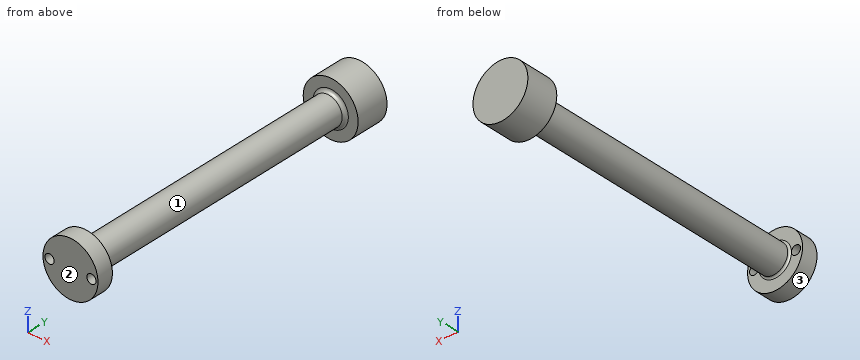
from build123d import *

# Parameters (mm, degrees)
SKETCH2_R          = 1.7779999999999996
CUT_EXTRUDE1_DEPTH = 6.35
FILLET1_R          = 1.27
FILLET2_R          = 0.762


with BuildPart() as part:
    # Sketch1 → Revolve1 (revolve)
    with BuildSketch(Plane.XY, mode=Mode.PRIVATE) as revolve1_sk:
        Polygon((0, 0), (10.668, 0), (10.668000000000001, 6.35), (5.588, 6.349999999999999), (5.588, 114.30000000000001), (10.668000000000001, 114.3), (10.668, 127), (-1.12e-14, 127), align=None)
    revolve(revolve1_sk.sketch.rotate(Axis((-1.12e-14, 127, 0), (9e-17, -1, 0)), 180), axis=Axis((-1.12e-14, 127, 0), (9e-17, -1, 0)))

    # Sketch2 → Cut-Extrude1 (cut)
    with BuildSketch(Plane(origin=(-5.6e-16, 6.349999999999999, 0), x_dir=(1, -1.7e-16, 0), z_dir=(1.7e-16, 1, 0))):
        with Locations(Location((-8.128000000000021, -4.5e-16, 0), (0, 0, 180))):
            Circle(SKETCH2_R)
        with Locations(Location((8.128000000000021, -4.5e-16, 0), (0, 0, 180))):
            Circle(SKETCH2_R)
    extrude(amount=-CUT_EXTRUDE1_DEPTH, mode=Mode.SUBTRACT)

    # Fillet1
    fillet1_edges = [part.edges().sort_by_distance(p)[0] for p in [
        (5.588000000000001, 114.30000000000001, -1.37e-15),
    ]]
    fillet(fillet1_edges, radius=FILLET1_R)

    # Fillet2
    fillet2_edges = [part.edges().sort_by_distance(p)[0] for p in [
        (5.587999999999999, 6.349999999999995, -3.85e-15),
    ]]
    fillet(fillet2_edges, radius=FILLET2_R)


solid = part.part
Could you check a few things on this model? Use its own coordinates, in mm. Face numbers are marked on the shaded views. Coordinates: 2 decimals unless noted, no trailing zeros. Order: outer loops, then holes, each group sorted by start corner. A loop starts at its lowest first (then second) coordinate and runs counter-clockwise, first axis right, second up. Notation, with made-up numbers: (10.25, 69) - (25.25, 69) arc R20 ccw to (25.25, 75) - close; hole circle Ø10 at (8.5, 48). An arc over 180 degrees is marked (long way). Answer in a Markdown table with one row per item. Add a question column.
(1) Will these pins go through, and if not, where does the flat tip stop? pin 1 (10 mm diameter, centred on x = 8.5, z = 0.5, fed in from -Y); pin 2 (10 mm diameter, centred on x = -2, y = 51, fed in from +Z); pin 3 (3 mm diameter, centred on x = -8.128, z = 0, fed in from -Y); pin 4 (10 mm diameter, centred on x = 6, y = 106, fed in from +Z).
(2) I need wall thicknesses on L1, parallel to Y at x = -0.5, z = -9; L2, parallel to Z at x = 1.5, y = 87; L3, parallel to Y at x = -6, z = 0.5. Which ranges of each line are inside material? Lowest first, please.
(3) If we section it at A-A, the plane x = 0: Please give me the cut outline in (y, z), then the cut area to 3 significant figures.
(4) If we section it at B-B, the plane z = -8.25: Please give me the cut outline in (x, y).
(5) If we mould it in two halves opening along Y, with no side actions, what happens to the marked faces 1, 2 and 3? For each: released by +Y, released by -Y, zero draft, split by the parting line, or undercut.
(6) If we section it at D-D, the plane z = 9: Please give me the cut outline in (x, y), then the cut area to 3 significant figures.
(7) If we section it at C-C, the plane y = 99: Please give me the cut outline in (x, z).
Results are:
| question | item | result |
|---|---|---|
| 1 | pin 1 | stops at y = 0 |
| 1 | pin 2 | stops at z = 5.59 |
| 1 | pin 3 | stops at y = 114.28 |
| 1 | pin 4 | stops at z = 5.5 |
| 2 | L1 | y = 0 to 6.35, 114.3 to 127 |
| 2 | L2 | z = -5.38 to 5.38 |
| 2 | L3 | y = 0 to 6.42, 113.98 to 127 |
| 3 | outline | (0, -10.67) - (6.35, -10.67) - (6.35, -6.35) arc R0.76 cw to (7.11, -5.59) - (113.03, -5.59) arc R1.27 cw to (114.3, -6.86) - (114.3, -10.67) - (127, -10.67) - (127, 10.67) - (114.3, 10.67) - (114.3, 6.86) arc R1.27 cw to (113.03, 5.59) - (7.11, 5.59) arc R0.76 cw to (6.35, 6.35) - (6.35, 10.67) - (0, 10.67) - close |
| 3 | area | 1,610 mm2 |
| 4 | outline | (-6.76, 0) - (6.76, 0) - (6.76, 6.35) - (-6.76, 6.35) - close; (-6.76, 114.3) - (6.76, 114.3) - (6.76, 127) - (-6.76, 127) - close |
| 5 | face 1 | undercut |
| 5 | face 2 | released by -Y |
| 5 | face 3 | zero draft |
| 6 | outline | (-5.73, 0) - (5.73, 0) - (5.73, 6.35) - (-5.73, 6.35) - close; (-5.73, 114.3) - (5.73, 114.3) - (5.73, 127) - (-5.73, 127) - close |
| 6 | area | 218 mm2 |
| 7 | outline | circle Ø11.18 at (0, 0) |
